from build123d import *

# Parameters (mm, degrees)
CROQUIS1_R              = 35
SALIENTE_EXTRUIR1_DEPTH = 15
CROQUIS2_R              = 8.5
CORTAR_EXTRUIR1_DEPTH   = 52.720402164
VACIADO1_T              = -2
REDONDEO1_R             = 2
REDONDEO2_R             = 4
CORTAR_EXTRUIR2_START   = -25
CORTAR_EXTRUIR2_DEPTH   = 27.720402164


with BuildPart() as part:
    # Croquis1 → Saliente-Extruir1 (new body)
    with BuildSketch(Plane.XY):
        Circle(CROQUIS1_R)
    extrude(amount=SALIENTE_EXTRUIR1_DEPTH)

    # Croquis2 → Cortar-Extruir1 (cut, through all)
    with BuildSketch(Plane.XY.offset(15)):
        Circle(CROQUIS2_R)
    extrude(amount=-CORTAR_EXTRUIR1_DEPTH, mode=Mode.SUBTRACT)

    # Vaciado1
    vaciado1_openings = [part.faces().sort_by_distance(p)[0] for p in [
        (-34.010050506, 0, 15),
    ]]
    offset(amount=VACIADO1_T, openings=vaciado1_openings, kind=Kind.INTERSECTION)

    # Redondeo1
    redondeo1_edges = [part.edges().sort_by_distance(p)[0] for p in [
        (-33, 0, 2),
        (-10.5, 0, 2),
    ]]
    fillet(redondeo1_edges, radius=REDONDEO1_R)

    # Redondeo2
    redondeo2_edges = [part.edges().sort_by_distance(p)[0] for p in [
        (-35, 0, 0),
    ]]
    fillet(redondeo2_edges, radius=REDONDEO2_R)

    # Croquis3 → Cortar-Extruir2 (cut, through all)
    with BuildSketch(Plane(origin=(0, 0, 0), x_dir=(1, 0, 0), z_dir=(0, 1, 0)).offset(CORTAR_EXTRUIR2_START)):
        with BuildLine():
            Line((-5, -2), (5, -2))
            ThreePointArc((5, -2), (7, -4), (5, -6))
            Line((5, -6), (-5, -6))
            ThreePointArc((-5, -6), (-7, -4), (-5, -2))
        make_face()
    extrude(amount=-CORTAR_EXTRUIR2_DEPTH, mode=Mode.SUBTRACT)


solid = part.part
Read the model definition and answer for the solid it produces. Units are mm, in the model's axes. A direction names the side the tool comes from. Round coordinates to 2 decimals unless told otherwise and drop trailing zeros. Order: outer loops, then holes, each group sorted by start corner. A loop starts at its lowest first (then second) coordinate and runs counter-clockwise, first axis right, second up.
1) Straight lines are drawn through the part: L1, parallel to Y at x = 0, z = 11.25; L2, parallel to Z at x = -6, y = 15.5; L3, parallel to X at y = -17, z = 3. For each, find the intervals that lie inside material, in ascending order.
2) The mould has two halves that part along Y. Classify faces 4 (the face through (0, 13, 2)), 5 (the face through (9, 0, 15)), 6 (the face through (-28, -21, 9)): released by +Y, released by -Y, zero draft, split by the parting line, or undercut.
3) For faces 1 (the face through (0, -34, 6)), 2 (the face through (6.5, -6.5, 0)), 3 (the face through (30.5, -12.6, 9.4)), determine the directions among +Z, -Z, +X, -X, +Y, -Y from which every point of the face is accessible in a straight line to the end or side of a thin tool.
4) Flat-ended cylindrical pins translate along their axes: pin 1 (10 mm diameter, centred on x = 0, y = 0, fed in from +Z); pin 2 (1 mm diameter, centred on y = 8.5, z = 3.5, fed in from -X); pin 3 (1 mm diameter, centred on y = 11.5, z = 2, fed in from -X); pin 4 (5 mm diameter, centred on x = -12, z = 7.5, fed in from +Y). Find the tip coordinate at first contact, or state that the pin passes through.
5) The part is cut by section C-C on z = 9.25. Write down the section's boundary in (x, y).
6) The part is cut by section A-A on y = 0. Write down the section's boundary in (x, z).
7) The part is cut by section B-B on x = 0. Write down the section's boundary in (y, z), plus the area to 3 significant figures.
Resolved:
1. L1: y = -35 to -33, -10.5 to -8.5, 8.5 to 10.5, 33 to 35
1. L2: z = 0 to 2
1. L3: x = -30.45 to -27.97, 27.97 to 30.45
2. face 4: undercut
2. face 5: zero draft
2. face 6: split by the parting line
3. face 1: -Y
3. face 2: -Z, +X, -X, +Y, -Y
3. face 3: +Z
4. pin 1: passes through
4. pin 2: stops at x = -34.05
4. pin 3: stops at x = -32.81
4. pin 4: stops at y = 33.69
5. outline: circle Ø70 at (0, 0); circle Ø21 at (0, 0); hole circle Ø66 at (0, 0); hole circle Ø17 at (0, 0)
6. outline: (-35, 4) arc R4 ccw to (-31, 0) - (-8.5, 0) - (-8.5, 15) - (-10.5, 15) - (-10.5, 4) arc R2 cw to (-12.5, 2) - (-31, 2) arc R2 cw to (-33, 4) - (-33, 15) - (-35, 15) - close; (8.5, 0) - (31, 0) arc R4 ccw to (35, 4) - (35, 15) - (33, 15) - (33, 4) arc R2 cw to (31, 2) - (12.5, 2) arc R2 cw to (10.5, 4) - (10.5, 15) - (8.5, 15) - close
7. outline: (-35, 6) - (-33, 6) - (-33, 15) - (-35, 15) - close; (-34.46, 2) arc R4 ccw to (-31, 0) - (-8.5, 0) - (-8.5, 15) - (-10.5, 15) - (-10.5, 4) arc R2 cw to (-12.5, 2) - close; (8.5, 0) - (31, 0) arc R4 ccw to (35, 4) - (35, 15) - (33, 15) - (33, 4) arc R2 cw to (31, 2) - (12.5, 2) arc R2 cw to (10.5, 4) - (10.5, 15) - (8.5, 15) - close
7. area: 198 mm2
